```python
from build123d import *

# Parameters (mm, degrees)
F0_W           = 385.6
F0_H           = 254
F1_DEPTH       = 10
F2_W           = 377
F2_H           = 222.3
F3_DEPTH       = 106.5
F5_D           = 6
F5_DEPTH       = 10
F5_TIP         = 1.8025818571
F6_D           = 5.1
F6_DEPTH       = 10
F6_CBORE_D     = 9
F6_CBORE_DEPTH = 5
F6_TIP         = 1.5321945785
F9_DEPTH       = 22.55
F10_R          = 8
F11_DEPTH      = 164.55
F12_R          = 14
F13_DEPTH      = 12


with BuildPart() as f1:
    # F0 (on Top) → F1 (new body)
    with BuildSketch(Plane.XY):
        Rectangle(F0_W, F0_H)
    extrude(amount=F1_DEPTH)

    # F2 (on face) → F3 (join)
    with BuildSketch(Plane(origin=(0, 0, 0), x_dir=(1, 0, 0), z_dir=(0, 0, -1))):
        Rectangle(F2_W, F2_H)
    extrude(amount=F3_DEPTH)

    # F5
    with Locations(Plane.XY.offset(10)):
        with Locations((-142.8, 115), (12.2, 115), (137.2, 115), (137.2, -115), (-17.8, -115), (-142.8, -115)):
            Hole(F5_D / 2, depth=F5_DEPTH)
            with Locations((0, 0, -(F5_DEPTH + F5_TIP / 2))):  # 118° drill point
                Cone(0, F5_D / 2, F5_TIP, mode=Mode.SUBTRACT)

    # F6
    with Locations(Plane.XY.offset(10)):
        with Locations((-174, 122), (-68, 122), (38, 122), (174, 122), (174, -122), (38, -122), (-68, -122), (-174, -122)):
            CounterBoreHole(F6_D / 2, F6_CBORE_D / 2, F6_CBORE_DEPTH, depth=F6_DEPTH)
            with Locations((0, 0, -(F6_DEPTH + F6_TIP / 2))):  # 118° drill point
                Cone(0, F6_D / 2, F6_TIP, mode=Mode.SUBTRACT)



with BuildPart() as f9:
    # F8 (on offset) → F9 (new body)
    with BuildSketch(Plane.XZ.offset(47.45)):
        with BuildLine():
            ThreePointArc((-81.0016359628, 162.7334830244), (-93.9756988655, 176.7052720437), (-110.6322861807, 167.4265169756))
            Line((-110.6322861807, 167.4265169756), (-139.90404485, -17.3880936599))
            Line((-139.90404485, -17.3880936599), (-110.2733946321, -22.0811276111))
            Line((-110.2733946321, -22.0811276111), (-81.0016359628, 162.7334830244))
        make_face()
    extrude(amount=F9_DEPTH)

    # F10 (on face) → F11 (join)
    with BuildSketch(Plane.XZ.offset(47.45)):
        with Locations((-95.8169610718, 165.08)):
            Circle(F10_R)
    extrude(amount=F11_DEPTH)

    # F12 (on face) → F13 (join)
    with BuildSketch(Plane.XZ.offset(212)):
        with Locations((-95.8169610718, 165.08)):
            Circle(F12_R)
    extrude(amount=-F13_DEPTH)


with BuildPart() as f1_1:
    add(f1.part)

    add(f9.part)  # F14 merges F9
    # F14: F9 across plane
    add(f9.part.mirror(Plane.XZ))


solid = f1_1.part
```
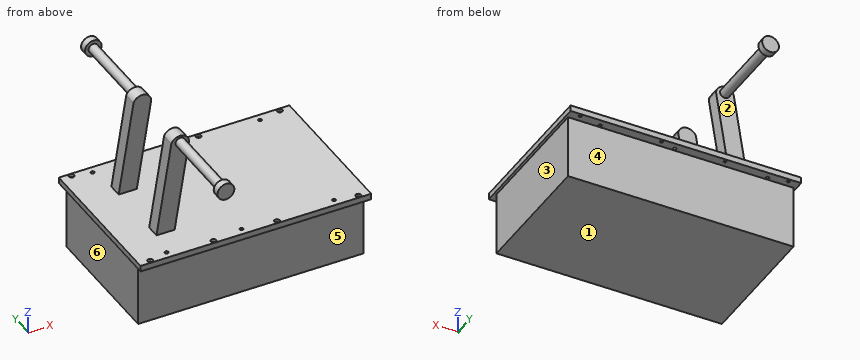
Geometry check sheet. Reference: the model listing, model coordinates, mm. Face numbers are marked on the shaded views. A direction names the side the tool comes from. Give positions to 0.01 mm unless a question says otherwise; leave off trailing zeros. Loops run counter-clockwise (first coordinate to the right, second up) from the corner with the lowest first, then second, coordinate; pieces in that order, holes last. Notation, with made-up numbers: M -5,85.5 L 26,85.5 A26 ccw 26,113.5 Z; hole C 1,79 d6. An arc over 180 degrees is marked long. Answer as CSV lines item,"result".
Item 1: Cross-section at C-C on y = -139.5. Record the cut outline in (x, z).
Values:
outline,"C -95.82,165.08 d16"
Item 2: Material ranges on line 1 (Y direction, x = 38, z = 6.5); line 2 (Y direction, x = -142.8, z = 3.5); line 3 (X direction, y = 115, z = 8.25), recorded low to high.
Values:
line 1,"y = -127 to -126.5, -117.5 to 117.5, 126.5 to 127"
line 2,"y = -127 to -118, -112 to 112, 118 to 127"
line 3,"x = -192.8 to -145.8, -139.8 to 9.2, 15.2 to 134.2, 140.2 to 192.8"
Item 3: Release check for a two-part mould opening along Z. For the marked faces 1, 2 and 3 record: pulls with the +Z half, pulls with the -Z half, needs draft (parallel to the pull), parting line crosses it, or undercut.
Values:
face 1,"pulls with the -Z half"
face 2,"undercut"
face 3,"needs draft"
Item 4: Cross-section at D-D on z = -21. Record the cut outline in (x, y), and give its area (3 significant figures).
Values:
outline,"M -188.5,-111.15 L 188.5,-111.15 L 188.5,111.15 L -188.5,111.15 Z"
area,"83,800 mm²"
Item 5: Access from +Z, -Z, +X, -X, +Y, -Y to the whole of each face (thin tool, end or side, straight path). Record for the marked faces 4, 5 and 6.
Values:
face 4,"-Z, +X, -X, +Y"
face 5,"-Z, +X, -X, -Y"
face 6,"-Z, -X, +Y, -Y"
Item 6: Depth check by flat-ended pin: P1, Ø8, axis at x = -91, z = 104, coming from the -Y side; P2, Ø2, axis at y = -52, z = 65, coming from the -X side; P3, Ø11, axis at x = 93.5, z = 7, coming from the +Y side. Enter the tip coordinate at first touch or a pass-through.
Values:
P1,"stops at y = -70"
P2,"stops at x = -127.01"
P3,"stops at y = 127"
Item 7: Cross-section at A-A on z = 142.5. Record the cut outline in (x, y), and give its area (3 significant figures).
Values:
outline,"M -114.58,-70 L -84.21,-70 L -84.21,-47.45 L -114.58,-47.45 Z; M -114.58,47.45 L -84.21,47.45 L -84.21,70 L -114.58,70 Z"
area,"1,370 mm²"
Item 8: Cross-section at B-B on x = 71.5. Record the cut outline in (y, z), and give its area (3 significant figures).
Values:
outline,"M -127,0 L -111.15,0 L -111.15,-106.5 L 111.15,-106.5 L 111.15,0 L 127,0 L 127,10 L -127,10 Z"
area,"26,200 mm²"
